```python
from build123d import *

# Parameters (mm, degrees)
F0_R       = 6
F1_DEPTH   = 4
F2_SIZE2   = 0.4
F2_SIZE    = 2
F2_2_SIZE2 = 0.4
F2_2_SIZE  = 2
F4_DEPTH   = 25
F6_DEPTH   = 1
F7_R       = 0.99999
F8_R       = 2.75
F9_DEPTH   = 0.2
F10_R      = 2.5
F11_DEPTH  = 25


# Not quite as in the source:
# - a fillet or chamfer is up to 0.001 mm smaller than in the source, because OpenCascade refuses the exact size


with BuildPart() as f1:
    # F0 (on Top) → F1 (new body)
    with BuildSketch(Plane.XY):
        Circle(F0_R)
    extrude(amount=F1_DEPTH)

    # F2
    f2_edges = [f1.edges().sort_by_distance(p)[0] for p in [
        (-6, 0, 4),
    ]]
    f2_side = f1.faces().sort_by_distance((0, 0, 4))[0]
    chamfer(f2_edges, length=F2_SIZE, length2=F2_SIZE2, reference=f2_side)

    # F2#2
    f2_2_edges = [f1.edges().sort_by_distance(p)[0] for p in [
        (-6, 0, 0),
    ]]
    f2_2_side = f1.faces().sort_by_distance((0, 0, 0))[0]
    chamfer(f2_2_edges, length=F2_2_SIZE, length2=F2_2_SIZE2, reference=f2_2_side)

    # F3 (on face) → F4 (intersect)
    with BuildSketch(Plane.XY.offset(4)):
        with BuildLine():
            Line((-4, -2.3094010768), (-1.9999999977, -3.4641016165))
            ThreePointArc((-1.9999999977, -3.4641016165), (-3.4641016145, -2.0000000012), (-4, 0))
            Line((-4, 0), (-4, -2.3094010768))
        make_face()
        with BuildLine():
            ThreePointArc((-4, 0), (-3.4641016358, 1.9999999642), (-2.0000000715, 3.4641015738))
            Line((-2.0000000715, 3.4641015738), (-4, 2.3094010768))
            Line((-4, 2.3094010768), (-4, 0))
        make_face()
        with BuildLine():
            ThreePointArc((-2.0000000715, 3.4641015738), (-2.18e-08, 4), (2.0000000338, 3.4641015956))
            Line((2.0000000338, 3.4641015956), (0, 4.6188021535))
            Line((0, 4.6188021535), (-2.0000000715, 3.4641015738))
        make_face()
        with BuildLine():
            Line((4, 0), (4, 2.3094010768))
            Line((4, 2.3094010768), (2.0000000338, 3.4641015956))
            ThreePointArc((2.0000000338, 3.4641015956), (3.4641016249, 1.9999999831), (4, 0))
        make_face()
        with BuildLine():
            Line((4, -2.3094010768), (4, 0))
            ThreePointArc((4, 0), (3.4641016169, -1.9999999969), (2.0000000062, -3.4641016116))
            Line((2.0000000062, -3.4641016116), (4, -2.3094010768))
        make_face()
        with BuildLine():
            Line((0, -4.6188021535), (2.0000000062, -3.4641016116))
            ThreePointArc((2.0000000062, -3.4641016116), (4.9e-09, -4), (-1.9999999977, -3.4641016165))
            Line((-1.9999999977, -3.4641016165), (0, -4.6188021535))
        make_face()
        with BuildLine():
            ThreePointArc((2.0000000062, -3.4641016116), (3.4641016169, -1.9999999969), (4, 0))
            ThreePointArc((4, 0), (3.4641016249, 1.9999999831), (2.0000000338, 3.4641015956))
            ThreePointArc((2.0000000338, 3.4641015956), (-2.18e-08, 4), (-2.0000000715, 3.4641015738))
            ThreePointArc((-2.0000000715, 3.4641015738), (-3.4641016358, 1.9999999642), (-4, 0))
            ThreePointArc((-4, 0), (-3.4641016145, -2.0000000012), (-1.9999999977, -3.4641016165))
            ThreePointArc((-1.9999999977, -3.4641016165), (4.9e-09, -4), (2.0000000062, -3.4641016116))
        make_face()
    extrude(amount=-F4_DEPTH, mode=Mode.INTERSECT)

    # F5 (on face) → F6 (join)
    with BuildSketch(Plane.XY.offset(4)):
        with BuildLine():
            ThreePointArc((1.9999999952, -3.4641016179), (3.4641016138, -2.0000000024), (4, 0))
            ThreePointArc((4, 0), (3.4641016188, 1.9999999936), (2.0000000128, 3.4641016077))
            ThreePointArc((2.0000000128, 3.4641016077), (0, 4), (-2.0000000128, 3.4641016077))
            ThreePointArc((-2.0000000128, 3.4641016077), (-3.4641016188, 1.9999999936), (-4, 0))
            ThreePointArc((-4, 0), (-3.4641016204, -1.9999999909), (-2.0000000181, -3.4641016047))
            ThreePointArc((-2.0000000181, -3.4641016047), (-1.32e-08, -4), (1.9999999952, -3.4641016179))
        make_face()
    extrude(amount=F6_DEPTH)

    # F7 (radius 1 in the source; OpenCascade refuses exactly that, so slightly less here)
    f7_edges = [f1.edges().sort_by_distance(p)[0] for p in [
        (-4, 0, 5),
    ]]
    fillet(f7_edges, radius=F7_R)

    # F8 (on face) → F9 (cut)
    with BuildSketch(Plane.XY.offset(5)):
        Circle(F8_R)
    extrude(amount=-F9_DEPTH, mode=Mode.SUBTRACT)

    # F10 (on face) → F11 (cut)
    with BuildSketch(Plane.XY.offset(4.8)):
        Circle(F10_R)
    extrude(amount=-F11_DEPTH, mode=Mode.SUBTRACT)


solid = f1.part
```
Model file for the job. Use its own axes, mm. Give positions to 0.01 mm unless a question says otherwise; leave off trailing zeros. Loops run counter-clockwise (first coordinate to the right, second up) from the corner with the lowest first, then second, coordinate; pieces in that order, holes last. Notation, with made-up numbers: (-14.75, 34) - (-0.75, 34) arc R10 ccw to (-0.75, 38) - close; hole circle Ø1 at (29, 0.25). An arc over 180 degrees is marked (long way). One line per item, written item: value. Start each with the question number.
1. Pull direction Y, two halves, no side cores. Call faces 1 (the conical face through (3.59, -2.08, 0.03)), 2 (the cylindrical face through (-0.54, -2.44, 2.43)), 3 (the conical face through (-3.59, 2.08, 0.03)): pulls with the +Y half, pulls with the -Y half, needs draft (parallel to the pull), parting line crosses it, or undercut.
2. Probe L1, parallel to X at y = -2, z = 0.75; L2, parallel to Y at x = -0.75, z = 3.15; L3, parallel to Z at x = 1.75, y = -2.5. List the from-to ranges inside material, lowest first. Write a range as from..to.
3. Slice it at B-B (z = 4.5). List the corners of the cut face in (x, y), plus the area to 3 significant figures.
4. Pin check, flat tip, straight feed: pin 1 (1.5 mm diameter, centred on x = -1, z = 1, fed in from -Y). Stop position of the tip, or through.
5. Slice it at A-A (z = 1.9). List the corners of the cut face in (x, y), plus the area to 3 significant figures.
Solution:
1. face 1: pulls with the -Y half
1. face 2: undercut
1. face 3: pulls with the +Y half
2. L1: x = -4..-1.5, 1.5..4
2. L2: y = -4.19..-2.38, 2.38..4.19
2. L3: z = 0..5
3. outline: circle Ø7.73 at (0, 0); hole circle Ø5 at (0, 0)
3. area: 27.3 mm^2
4. pin 1: stops at y = -4.47
5. outline: (-4, -2.31) - (0, -4.62) - (4, -2.31) - (4, 2.31) - (0, 4.62) - (-4, 2.31) - close; hole circle Ø5 at (0, 0)
5. area: 35.8 mm^2
